Autodesk Inventor part; units mm, degrees
ref_plane "YZ Plane" through (0, 0, 0) normal (1, 0, 0) x (0, 1, 0)
ref_plane "XZ Plane" through (0, 0, 0) normal (0, 1, 0) x (-1, 0, 0)
ref_plane "XY Plane" through (0, 0, 0) normal (0, 0, 1) x (1, 0, 0)
sketch "Sketch1" plane through (0, 0, 0) normal (0, 0, 1) x (1, 0, 0)
  line L0 (-110, -75) -> (110, -75)
  line L1 (110, -75) -> (110, 75)
  line L2 (110, 75) -> (-110, 75)
  line L3 (-110, 75) -> (-110, -75)
  line L4 (-110, -75) -> (110, 75) construction
  line L5 (110, -75) -> (-110, 75) construction
  point P0 (0, 0)
  dimension "d0" = 220
  dimension "d1" = 150
extrude "Extrusion1" add sketch "Sketch1" along normal blind 5
sketch "Sketch2" plane through (0, 0, 0) normal (0, 0, -1) x (-1, 0, 0)
  circle A0 centre (100, 15) radius 2
  circle A1 centre (-100, -65) radius 2
  circle A2 centre (100, -65) radius 2
  circle A3 centre (-100, 15) radius 2
  line L0 (-110, -75) -> (-80, -75)
  line L1 (-80, -75) -> (-80, -70)
  line L2 (-95, -70) -> (-80, -70)
  line L3 (-95, -70) -> (-95, -60)
  line L4 (-95, -60) -> (-105, -60)
  line L5 (-105, -60) -> (-105, 10)
  line L6 (-105, 10) -> (-95, 10)
  line L7 (-95, 10) -> (-95, 20)
  line L8 (-95, 20) -> (-105, 20)
  line L9 (-105, 20) -> (-105, 25)
  arc A4 (-60, 70) -> (-105, 25) centre (-60, 25) ccw
  line L10 (-60, 70) -> (60, 70)
  arc A5 (105, 25) -> (60, 70) centre (60, 25) ccw
  line L11 (105, 20) -> (105, 25)
  line L12 (105, 20) -> (95, 20)
  line L13 (95, 20) -> (95, 10)
  line L14 (95, 10) -> (105, 10)
  line L15 (105, -60) -> (105, 10)
  line L16 (105, -60) -> (95, -60)
  line L17 (95, -60) -> (95, -70)
  line L18 (80, -70) -> (95, -70)
  line L19 (80, -70) -> (80, -75)
  line L20 (80, -75) -> (110, -75)
  line L21 (110, -75) -> (110, 25)
  arc A6 (110, 25) -> (60, 75) centre (60, 25) ccw
  line L22 (-60, 75) -> (60, 75)
  arc A7 (-60, 75) -> (-110, 25) centre (-60, 25) ccw
  line L23 (-110, -75) -> (-110, 25)
  line L24 (-110, -75) -> (110, -75)
  line L25 (110, -75) -> (110, 75)
  line L26 (110, 75) -> (-110, 75)
  line L27 (-110, 75) -> (-110, -75)
  line L28 (-110, -75) -> (110, 75) construction
  line L29 (110, -75) -> (-110, 75) construction
  point P0 (0, 0)
  point P1 (-110, 25)
extrude "Extrusion2" cut sketch "Sketch2" against normal blind 5 contours A0 | A1 | A2 | A3 | L27 L26 A7 | L26 L25 A6
sketch "Sketch4" plane through (0, 0, 0) normal (0, 0, -1) x (-1, 0, 0)
  line L0 (-55, -75) -> (55, -75)
  line L1 (55, -75) -> (55, 15)
  line L2 (35, 35) -> (-35, 35)
  line L3 (-55, 15) -> (-55, -75)
  line L4 (110, -75) -> (-110, -75)
  arc A0 (-35, 35) -> (-55, 15) centre (-35, 15) ccw
  arc A1 (55, 15) -> (35, 35) centre (35, 15) ccw
  point P0 (0, 0)
  point P1 (55, 35)
  point P2 (-55, 35)
  dimension "d12" = 110
  dimension "d13" = 110
  dimension "d14" = 55
  dimension "d15" = 20
extrude "Extrusion4" cut sketch "Sketch4" against normal blind 5
properties part number "speaker_front" material "ABS Plastic"
Here's how the part is built. I have some questions about the finished solid (model axes, mm). A direction names the side the tool comes from. Coordinates: 2 decimals unless noted, no trailing zeros. Loops run counter-clockwise (first coordinate to the right, second up) from the corner with the lowest first, then second, coordinate; pieces in that order, holes last.
1. Imagine slicing it at A-A, the plane y = -51. Please give me the cut outline in (x, z).
2. If we mould it in two halves opening along Y, with no side actions, what happens to faces 1 (the flat face through (-2, 51, 0)), 2 (the cylindrical face through (-101.908, 15.601, 2.465)), 3 (the flat face through (82, -75, 2)), 4 (the cylindrical face through (98.092, 15.601, 2.465))? For each: pulls with the +Y half, pulls with the -Y half, needs draft (parallel to the pull), parting line crosses it, or undercut.
3. Imagine slicing it at C-C, the plane x = 27.5. Please give me the cut outline in (y, z).
4. Imagine slicing it at D-D, the plane y = 64. Please give me the cut outline in (x, z), and give its area (3 significant figures).
5. I need wall thicknesses on L1, parallel to Y at x = -100, z = 1.4; L2, parallel to X at y = -3, z = 2.85; L3, parallel to Y at x = 17.5, z = 0.4. Which ranges of each line are inside material? Lowest first, please.
6. For P1, Ø5, axis at x = 100, y = 15, coming from the +Z side; P2, Ø3, axis at x = 100, y = -65, coming from the +Z side, each with a flat end and sliding along its axis, tell me the tip position at first contact or that it passes through.
7. For faces 5 (the cylindrical face through (98.925, -63.314, 2.465)), 6 (the flat face through (55, -29, 2)), which set-ups out of +Z, -Z, +X, -X, +Y, -Y let a thin tool reach every point of the face, with its end or its side?
8. Imagine slicing it at B-B, the plane z = 2.65. Please give me the cut outline in (x, y).
Taken from the geometry:
1. outline: (-110, 0) - (-55, 0) - (-55, 5) - (-110, 5) - close; (55, 0) - (110, 0) - (110, 5) - (55, 5) - close
2. face 1: needs draft
2. face 2: undercut
2. face 3: pulls with the -Y half
2. face 4: undercut
3. outline: (35, 0) - (75, 0) - (75, 5) - (35, 5) - close
4. outline: (-91.29, 0) - (91.29, 0) - (91.29, 5) - (-91.29, 5) - close
4. area: 913 mm2
5. L1: y = -75 to -67, -63 to 13, 17 to 55
5. L2: x = -110 to -55, 55 to 110
5. L3: y = 35 to 75
6. P1: stops at z = 5
6. P2: passes through
7. face 5: +Z, -Z
7. face 6: +Z, -Z, -Y
8. outline: (-110, -75) - (-55, -75) - (-55, 15) arc R20 cw to (-35, 35) - (35, 35) arc R20 cw to (55, 15) - (55, -75) - (110, -75) - (110, 25) arc R50 ccw to (60, 75) - (-60, 75) arc R50 ccw to (-110, 25) - close; hole circle Ø4 at (-100, -65); hole circle Ø4 at (-100, 15); hole circle Ø4 at (100, -65); hole circle Ø4 at (100, 15)
